```python
from build123d import *

# Parameters (mm, degrees)
SCHIZZO1_W                   = 141.6
SCHIZZO1_H                   = 41.6
ESTRUSIONE_ESTRUSIONE1_DEPTH = 28
ESTRUSIONE_ESTRUSIONE2_DEPTH = 0.5


with BuildPart() as part:
    # Schizzo1 → Estrusione-Estrusione1 (new body)
    with BuildSketch(Plane(origin=(0, 0, 0), x_dir=(1, 0, 0), z_dir=(0, 1, 0))):
        Rectangle(SCHIZZO1_W, SCHIZZO1_H)
    extrude(amount=ESTRUSIONE_ESTRUSIONE1_DEPTH)

    # Schizzo2 → Estrusione-Estrusione2 (add)
    with BuildSketch(Plane(origin=(0, 0, 0), x_dir=(1, 0, 0), z_dir=(0, 1, 0))):
        with BuildLine():
            Line((-70.8, 20.8), (-70.8, 28))
            ThreePointArc((-70.8, 28), (-70.214213562, 29.414213562), (-68.8, 30))
            Line((-68.8, 30), (-67.3, 30))
            Line((-67.3, 30), (-67.3, 25.8))
            ThreePointArc((-67.3, 25.8), (-65.3, 23.8), (-63.3, 25.8))
            Line((-63.3, 25.8), (-63.3, 30))
            Line((-63.3, 30), (-61.8, 30))
            ThreePointArc((-61.8, 30), (-60.385786438, 29.414213562), (-59.8, 28))
            Line((-59.8, 28), (-59.8, 20.8))
            Line((-59.8, 20.8), (-70.8, 20.8))
        make_face()
        with BuildLine():
            Line((-63.3, -30), (-61.8, -30))
            ThreePointArc((-61.8, -30), (-60.385786438, -29.414213562), (-59.8, -28))
            Line((-59.8, -28), (-59.8, -20.8))
            Line((-59.8, -20.8), (-70.8, -20.8))
            Line((-70.8, -20.8), (-70.8, -28))
            ThreePointArc((-70.8, -28), (-70.214213562, -29.414213562), (-68.8, -30))
            Line((-68.8, -30), (-67.3, -30))
            Line((-67.3, -30), (-67.3, -25.8))
            ThreePointArc((-67.3, -25.8), (-65.3, -23.8), (-63.3, -25.8))
            Line((-63.3, -25.8), (-63.3, -30))
        make_face()
        with BuildLine():
            Line((63.3, -30), (61.8, -30))
            ThreePointArc((61.8, -30), (60.385786438, -29.414213562), (59.8, -28))
            Line((59.8, -28), (59.8, -20.8))
            Line((59.8, -20.8), (70.8, -20.8))
            Line((70.8, -20.8), (70.8, -28))
            ThreePointArc((70.8, -28), (70.214213562, -29.414213562), (68.8, -30))
            Line((68.8, -30), (67.3, -30))
            Line((67.3, -30), (67.3, -25.8))
            ThreePointArc((67.3, -25.8), (65.3, -23.8), (63.3, -25.8))
            Line((63.3, -25.8), (63.3, -30))
        make_face()
        with BuildLine():
            Line((63.3, 30), (61.8, 30))
            ThreePointArc((61.8, 30), (60.385786438, 29.414213562), (59.8, 28))
            Line((59.8, 28), (59.8, 20.8))
            Line((59.8, 20.8), (70.8, 20.8))
            Line((70.8, 20.8), (70.8, 28))
            ThreePointArc((70.8, 28), (70.214213562, 29.414213562), (68.8, 30))
            Line((68.8, 30), (67.3, 30))
            Line((67.3, 30), (67.3, 25.8))
            ThreePointArc((67.3, 25.8), (65.3, 23.8), (63.3, 25.8))
            Line((63.3, 25.8), (63.3, 30))
        make_face()
    extrude(amount=ESTRUSIONE_ESTRUSIONE2_DEPTH)


solid = part.part
```
Geometry check sheet. Reference: the model listing, model coordinates, mm. A direction names the side the tool comes from. Give positions to 0.01 mm unless a question says otherwise; leave off trailing zeros. Write each loop counter-clockwise with the first axis right and the second up, starting at its lowest first coordinate (ties: lowest second). Pieces come first, ordered by that corner, then holes.
1) Section check A-A, the plane x = -65.3. Record the boundary of the cut face in (y, z).
2) Section check C-C, the plane x = 54.5. Record the boundary of the cut face in (y, z).
3) Gauge pin test, flat ends, axial feed: pin 1 (10 mm diameter, centred on x = -5.5, y = 12, fed in from -Z); pin 2 (0.6 mm diameter, centred on y = 0, z = -28.5, fed in from -X); pin 3 (10 mm diameter, centred on x = -63.5, z = -26.5, fed in from +Y). Record the tip position at first contact, or that the pin passes through.
4) Section check B-B, the plane y = 6. Record the boundary of the cut face in (x, z).
5) Material ranges on L1, parallel to Z at x = 21, y = 7, recorded low to high.
6) Access from +Z, -Z, +X, -X, +Y, -Y to the whole of each face (thin tool, end or side, straight path). Record for faces 1 (the flat face through (65, 0.5, 23)), 2 (the flat face through (-70.8, 14, 0)), 3 (the flat face through (-65, 0.5, -23)).
Computed:
1. outline: (0, -23.8) - (0.5, -23.8) - (0.5, -20.8) - (28, -20.8) - (28, 20.8) - (0.5, 20.8) - (0.5, 23.8) - (0, 23.8) - close
2. outline: (0, -20.8) - (28, -20.8) - (28, 20.8) - (0, 20.8) - close
3. pin 1: stops at z = -20.8
3. pin 2: stops at x = -70.79
3. pin 3: stops at y = 0.5
4. outline: (-70.8, -20.8) - (70.8, -20.8) - (70.8, 20.8) - (-70.8, 20.8) - close
5. L1: z = -20.8 to 20.8
6. face 1: +Z, +X, -X, +Y
6. face 2: +Z, -Z, -X, +Y, -Y
6. face 3: -Z, +X, -X, +Y
